Check sheet for the modelled part. Datum: model origin and axes. Units: mm. A direction names the side the tool comes from. Round coordinates to 2 decimals unless told otherwise and drop trailing zeros. Write each loop counter-clockwise with the first axis right and the second up, starting at its lowest first coordinate (ties: lowest second). Pieces come first, ordered by that corner, then holes.
Item 1: Section check A-A, the plane x = 0. Record the cut outline in (y, z), plus the area to 3 significant figures.
Item 2: Depth check by flat-ended pin: pin 1 (6 mm diameter, centred on x = -0.5, y = 1.5, fed in from -Z); pin 2 (3 mm diameter, centred on y = -7.5, z = 3.5, fed in from -X); pin 3 (2 mm diameter, centred on x = 8.5, z = 3, fed in from -Y). Enter the tip coordinate at first touch or a pass-through.
Item 3: Section check C-C, the plane y = -1. Record the cut outline in (x, z).
Item 4: Set-up check for faces 1 (the flat face through (0, 5.75, 2)), 2 (the cylindrical face through (-2.579, -1.978, 5.76)): record each of +Z, -Z, +X, -X, +Y, -Y from which the full face is reachable in a straight line by a thin tool's end or side.
Item 5: Material ranges on line 1 along Y through (x, z) = (0, 6.2); line 2 along X through (y, z) = (3, 4.75); line 3 along Y through (x, z) = (8.5, 2), recorded low to high.
Item 6: Release check for a two-part mould opening along X. For faces 3 (the flat face through (3, 3, 5)), 4 (the flat face through (6, -3, 0)) record: pulls with the +X half, pulls with the -X half, needs draft (parallel to the pull), parting line crosses it, or undercut.
Item 7: Section check B-B, the plane z = 4.25. Record the cut outline in (x, y), plus the area to 3 significant figures.
Item 8: Section check D-D, the plane x = 5.5. Record the cut outline in (y, z).
from build123d import *

# Parameters (mm, degrees)
F1_DEPTH = 6.5
F2_R     = 3.25
F3_DEPTH = 25
F5_DEPTH = 5


with BuildPart() as f1:
    # F0 (on Top) → F1 (new body)
    with BuildSketch(Plane.XY):
        with BuildLine():
            ThreePointArc((2.892627, 10.795431), (0, 13), (-2.892627, 10.795431))
            ThreePointArc((-2.892627, 10.795431), (-6.5, 11.25833), (-7.902804, 7.902804))
            ThreePointArc((-7.902804, 7.902804), (-11.25833, 6.5), (-10.795431, 2.892627))
            ThreePointArc((-10.795431, 2.892627), (-13, 0), (-10.795431, -2.892627))
            ThreePointArc((-10.795431, -2.892627), (-11.25833, -6.5), (-7.902804, -7.902804))
            ThreePointArc((-7.902804, -7.902804), (-6.5, -11.25833), (-2.892627, -10.795431))
            ThreePointArc((-2.892627, -10.795431), (0, -13), (2.892627, -10.795431))
            ThreePointArc((2.892627, -10.795431), (6.5, -11.25833), (7.902804, -7.902804))
            ThreePointArc((7.902804, -7.902804), (11.25833, -6.5), (10.795431, -2.892627))
            ThreePointArc((10.795431, -2.892627), (13, 0), (10.795431, 2.892627))
            ThreePointArc((10.795431, 2.892627), (11.25833, 6.5), (7.902804, 7.902804))
            ThreePointArc((7.902804, 7.902804), (6.5, 11.25833), (2.892627, 10.795431))
        make_face()
    extrude(amount=F1_DEPTH)

    # F2 (on face) → F3 (cut)
    with BuildSketch(Plane.XY.offset(6.5)):
        Circle(F2_R)
    extrude(amount=-F3_DEPTH, mode=Mode.SUBTRACT)

    # F4 (on Top) → F5 (cut)
    with BuildSketch(Plane.XY):
        Polygon((3.319764, 5.75), (-3.319764, 5.75), (-6.639528, 0), (-3.319764, -5.75), (3.319764, -5.75), (6.639528, 0), align=None)
    extrude(amount=F5_DEPTH, mode=Mode.SUBTRACT)


solid = f1.part
Values found:
1. outline: (-13, 0) - (-5.75, 0) - (-5.75, 5) - (-3.25, 5) - (-3.25, 6.5) - (-13, 6.5) - close; (3.25, 5) - (5.75, 5) - (5.75, 0) - (13, 0) - (13, 6.5) - (3.25, 6.5) - close
1. area: 102 mm2
2. pin 1: stops at z = 5
2. pin 2: stops at x = -11.49
2. pin 3: stops at y = -10.32
3. outline: (-12.83, 0) - (-6.06, 0) - (-6.06, 5) - (-3.09, 5) - (-3.09, 6.5) - (-12.83, 6.5) - close; (3.09, 5) - (6.06, 5) - (6.06, 0) - (12.83, 0) - (12.83, 6.5) - (3.09, 6.5) - close
4. face 1: -Z
4. face 2: +Z, -Z
5. line 1: y = -13 to -3.25, 3.25 to 13
5. line 2: x = -10.9 to -4.91, 4.91 to 10.9
5. line 3: y = -8 to 8
6. face 3: undercut
6. face 4: needs draft
7. outline: (-10.8, -2.89) arc R3 ccw to (-7.9, -7.9) arc R3 ccw to (-2.89, -10.8) arc R3 ccw to (2.89, -10.8) arc R3 ccw to (7.9, -7.9) arc R3 ccw to (10.8, -2.89) arc R3 ccw to (10.8, 2.89) arc R3 ccw to (7.9, 7.9) arc R3 ccw to (2.89, 10.8) arc R3 ccw to (-2.89, 10.8) arc R3 ccw to (-7.9, 7.9) arc R3 ccw to (-10.8, 2.89) arc R3 ccw to start; hole (-6.64, 0) - (-3.32, -5.75) - (3.32, -5.75) - (6.64, 0) - (3.32, 5.75) - (-3.32, 5.75) - close
7. area: 373 mm2
8. outline: (-11.62, 0) - (-1.97, 0) - (-1.97, 5) - (1.97, 5) - (1.97, 0) - (11.62, 0) - (11.62, 6.5) - (-11.62, 6.5) - close
